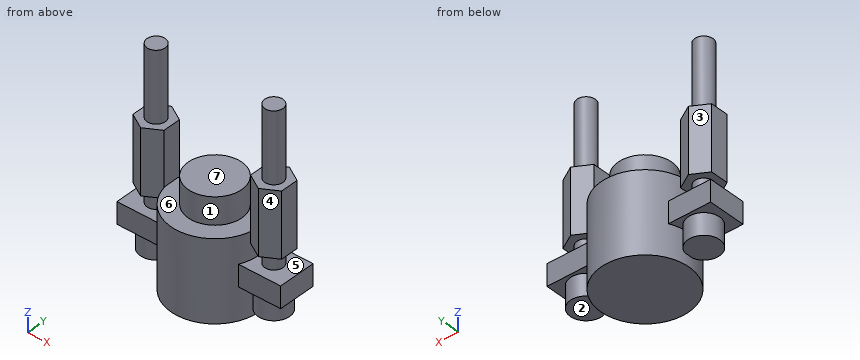
```python
from build123d import *

# Parameters (mm, degrees)
PRISM_DEPTH              = 12
CLONE139_PLACEMENT_ANGLE = 30
BOX251_W                 = 30.6
BOX251_H                 = 7
BOX251_DEPTH             = 4
CYLINDER_R               = 2.95
CYLINDER_DEPTH           = 7
CYLINDER001_R            = 1.7
CYLINDER001_DEPTH        = 30
CYLINDER1015_R           = 5
CYLINDER1015_DEPTH       = 10
CYLINDER1003_R           = 8.2
CYLINDER1003_DEPTH       = 15
CLONE140_PLACEMENT_ANGLE = 30


with BuildPart() as m3nut:
    # Prism → Prism (new body)
    with BuildSketch(Plane.XY):
        Polygon((3.35, 0), (1.675, 2.901185), (-1.675, 2.901185), (-3.35, 0), (-1.675, -2.901185), (1.675, -2.901185), align=None)
    extrude(amount=PRISM_DEPTH)


with BuildPart() as clone_of_m3nut005:
    # Clone139 base: copy of M3Nut
    add(m3nut.part)


with BuildPart() as clone_of_m3nut005_1:
    # Clone139 placement: moved
    add(clone_of_m3nut005.part.moved(Location((11, 0, 7))).rotate(Axis((11, 0, 7), (0, 0, 1)), CLONE139_PLACEMENT_ANGLE))


with BuildPart() as cube015:
    # Box251 → Box251 (new body)
    with BuildSketch(Plane(origin=(-15.3, -3.5, 0), x_dir=(1, 0, 0), z_dir=(0, 0, 1))):
        with Locations((15.3, 3.5)):
            Rectangle(BOX251_W, BOX251_H)
    extrude(amount=BOX251_DEPTH)


with BuildPart() as m3bolthead:
    # Cylinder → Cylinder (new body)
    with BuildSketch(Plane.XY):
        Circle(CYLINDER_R)
    extrude(amount=CYLINDER_DEPTH)


with BuildPart() as m3bolt:
    # Cylinder001 → Cylinder001 (new body)
    with BuildSketch(Plane.XY.offset(6)):
        Circle(CYLINDER001_R)
    extrude(amount=CYLINDER001_DEPTH)

    # Fusion: union M3BoltHead
    add(m3bolthead.part)


with BuildPart() as clone_of_m3bolt039:
    # Clone137 base: copy of M3Bolt
    add(m3bolt.part)


with BuildPart() as clone_of_m3bolt039_1:
    # Clone137 placement: moved
    add(clone_of_m3bolt039.part.moved(Location((11, 0, -4))))


with BuildPart() as clone_of_m3bolt040:
    # Clone138 base: copy of M3Bolt
    add(m3bolt.part)


with BuildPart() as clone_of_m3bolt040_1:
    # Clone138 placement: moved
    add(clone_of_m3bolt040.part.moved(Location((-11, 0, -4))))


with BuildPart() as cylinder021:
    # Cylinder1015 → Cylinder1015 (new body)
    with BuildSketch(Plane.XY.offset(4)):
        Circle(CYLINDER1015_R)
    extrude(amount=CYLINDER1015_DEPTH)


with BuildPart() as obj1:
    # Cylinder1003 → Cylinder1003 (new body)
    with BuildSketch(Plane.XY):
        Circle(CYLINDER1003_R)
    extrude(amount=CYLINDER1003_DEPTH)


with BuildPart() as obj1_1:
    # Clone136 placement: moved
    add(obj1.part.moved(Location((0, 0, -6))))


with BuildPart() as obj2:
    # Clone140 base: copy of M3Nut
    add(m3nut.part)


with BuildPart() as obj2_1:
    # Clone140 placement: moved
    add(obj2.part.moved(Location((-11, 0, 7))).rotate(Axis((-11, 0, 7), (0, 0, 1)), CLONE140_PLACEMENT_ANGLE))

    # Fusion062: union Clone of M3Nut005, Cube015, Clone of M3Bolt039, Clone of M3Bolt040, Cylinder021, obj1
    add(clone_of_m3nut005_1.part)
    add(cube015.part)
    add(clone_of_m3bolt039_1.part)
    add(clone_of_m3bolt040_1.part)
    add(cylinder021.part)
    add(obj1_1.part)


solid = obj2_1.part
```
Source: CAD feature listing. Evaluate the final solid. Frame: model axes, mm. Face numbers are marked on the shaded views. A direction names the side the tool comes from. Round coordinates to 2 decimals unless told otherwise and drop trailing zeros. Loops run counter-clockwise (first coordinate to the right, second up) from the corner with the lowest first, then second, coordinate; pieces in that order, holes last.
1. Section query C-C on y = 0. Give the number of separate pieces and of enclosed holes in the cut face, and give its area (3 significant figures).
2. Section query D-D on z = 3.5. Output: boundary loops of the cut face in (x, y).
3. Section query B-B on x = 0. Output: boundary loops of the cut face in (y, z).
4. Mould query, pull axis X, two halves, no side actions, for the marked faces 1, 2, 3 and 4. Classes: released by +X, released by -X, zero draft, split by the parting line, or undercut.
5. Contact query for flat-ended pins moving along their axis: pin 1 (1.7 mm diameter, centred on y = 0, z = 10.5, fed in from +X); pin 2 (6.5 mm diameter, centred on x = -11.5, y = -1, fed in from -Z); pin 3 (5 mm diameter, centred on y = -0.5, z = 8, fed in from -X); pin 4 (4.5 mm diameter, centred on x = 10, y = -0.5, fed in from -Z). Output: stop coordinate, or through.
6. Ray query, L1, parallel to X at y = 3, z = 11.5; L2, parallel to Z at x = 6.5, y = -3; L3, parallel to Z at x = -1, y = -3.75. Return the intervals inside material, ascending.
7. Section query A-A on z = 15. Output: boundary loops of the cut face in (x, y) (3 decimals).
8. Access query for the marked faces 5, 6 and 7. Directions: +Z, -Z, +X, -X, +Y, -Y. A direction counts if a zero-diameter tool reaches every point of the face in a straight line with its end or side. Return the directions, or none.
Answers below:
1. separate pieces: 1
1. enclosed holes: 2
1. area: 646 mm2
2. outline: (-15.3, -3.5) - (-7.42, -3.5) arc R8.2 ccw to (7.42, -3.5) - (15.3, -3.5) - (15.3, 3.5) - (7.42, 3.5) arc R8.2 ccw to (-7.42, 3.5) - (-15.3, 3.5) - close
3. outline: (-8.2, -6) - (8.2, -6) - (8.2, 9) - (5, 9) - (5, 14) - (-5, 14) - (-5, 9) - (-8.2, 9) - close
4. face 1: undercut
4. face 2: zero draft
4. face 3: released by -X
4. face 4: released by +X
5. pin 1: stops at x = 13.9
5. pin 2: stops at z = -4
5. pin 3: stops at x = -13.9
5. pin 4: stops at z = -6
6. L1: x = -11.61 to -10.39, -4 to 4, 10.39 to 11.61
6. L2: z = -6 to 9
6. L3: z = -6 to 14
7. outline: (-13.901, -1.675) - (-11, -3.35) - (-8.099, -1.675) - (-8.099, 1.675) - (-11, 3.35) - (-13.901, 1.675) - close; (8.099, -1.675) - (11, -3.35) - (13.901, -1.675) - (13.901, 1.675) - (11, 3.35) - (8.099, 1.675) - close
8. face 5: none
8. face 6: +Z
8. face 7: +Z, +Y, -Y
